Work out the finished part from the listing and answer in its coordinate system (mm). A direction names the side the tool comes from. Round coordinates to 2 decimals unless told otherwise and drop trailing zeros. Loops run counter-clockwise (first coordinate to the right, second up) from the corner with the lowest first, then second, coordinate; pieces in that order, holes last.
```python
from build123d import *

# Parameters (mm, degrees)
BASE_FLANGE1_DEPTH = 10
SKETCH6_R          = 2.5
CUT_EXTRUDE1_DEPTH = 35.932076949
SKETCH7_R          = 2
CUT_EXTRUDE2_DEPTH = 36.305806888


# Sheet-metal steps are written as plain solids
with BuildPart() as part:
    # Sketch1 → Base-Flange1 (new body)
    with BuildSketch(Plane.XY):
        with BuildLine():
            Line((0, 0), (13, 0))
            ThreePointArc((13, 0), (13.530330086, 0.219669914), (13.75, 0.75))
            Line((13.75, 0.75), (13.75, 5.75))
            ThreePointArc((13.75, 5.75), (14.409009742, 7.340990258), (16, 8))
            Line((16, 8), (32.5, 8))
            Line((32.5, 8), (32.5, 6.5))
            Line((32.5, 6.5), (16, 6.5))
            ThreePointArc((16, 6.5), (15.469669914, 6.280330086), (15.25, 5.75))
            Line((15.25, 5.75), (15.25, 0.75))
            ThreePointArc((15.25, 0.75), (14.590990258, -0.840990258), (13, -1.5))
            Line((13, -1.5), (0, -1.5))
            Line((0, -1.5), (0, 0))
        make_face()
    extrude(amount=BASE_FLANGE1_DEPTH)

    # Sketch6 → Cut-Extrude1 (cut, through all)
    with BuildSketch(Plane(origin=(0, 0, 0), x_dir=(1, 0, 0), z_dir=(0, 1, 0))):
        with Locations(Location((7.5, -5, 0), (0, 0, 270))):
            Circle(SKETCH6_R)
    extrude(amount=-CUT_EXTRUDE1_DEPTH, mode=Mode.SUBTRACT)

    # Sketch7 → Cut-Extrude2 (cut, through all)
    with BuildSketch(Plane(origin=(0, 8, 0), x_dir=(1, 0, 0), z_dir=(0, 1, 0))):
        with Locations(Location((27.5, -5, 0), (0, 0, 270))):
            Circle(SKETCH7_R)
    extrude(amount=-CUT_EXTRUDE2_DEPTH, mode=Mode.SUBTRACT)


solid = part.part
```
1. Consider probe 1 along Y at (x, z) = (9, 7.25); probe 2 along Y at (x, z) = (18.5, 0.5); probe 3 along X at (y, z) = (-0.5, 5). Determine where each line is inside the solid, lowest interval first.
Answer key:
probe 1: y = -1.5 to 0
probe 2: y = 6.5 to 8
probe 3: x = 0 to 5, 10 to 14.87
2. Determine the mould class of faces 1 (the face through (5.28, -0.74, 6.15)), 2 (the face through (15, 4, 10)), 3 (the face through (5, 0, 4)) for opening direction Z: +Z half, -Z half, draft (parallel to the pull), parting line (faces both ways), or undercut.
Answer key:
face 1: undercut
face 2: +Z half
face 3: draft
3. Find section A-A (z = 5). Write down the section's boundary in (x, y), then the cut area to 3 significant figures.
Answer key:
outline: (0, -1.5) - (5, -1.5) - (5, 0) - (0, 0) - close; (10, -1.5) - (13, -1.5) arc R2.25 ccw to (15.25, 0.75) - (15.25, 5.75) arc R0.75 cw to (16, 6.5) - (25.5, 6.5) - (25.5, 8) - (16, 8) arc R2.25 ccw to (13.75, 5.75) - (13.75, 0.75) arc R0.75 cw to (13, 0) - (10, 0) - close; (29.5, 6.5) - (32.5, 6.5) - (32.5, 8) - (29.5, 8) - close
area: 45.3 mm2
4. Given pin 1 (2 mm diameter, centred on y = 2.5, z = 6.5, fed in from -X); pin 2 (1 mm diameter, centred on y = 4.5, z = 8, fed in from +X); pin 3 (3 mm diameter, centred on x = 8.5, z = 3.5, fed in from +Y), each flat-ended and moving along its own axis, determine where each tip first touches the part or whether it passes through.
Answer key:
pin 1: stops at x = 13.75
pin 2: stops at x = 15.25
pin 3: stops at y = 0
5. Find section C-C (x = 24). Write down the section's boundary in (y, z), then the cut area to 3 significant figures.
Answer key:
outline: (6.5, 0) - (8, 0) - (8, 10) - (6.5, 10) - close
area: 15.0 mm2
6. Which of the six approach directions +Z, -Z, +X, -X, +Y, -Y give full straight-line access (tool end or side, diameter ignored) to faces 4 (the face through (24, 6.5, 5)), 5 (the face through (13.75, 3, 5)), 6 (the face through (0, -1, 5))?
Answer key:
face 4: +Z, -Z, +X, -Y
face 5: +Z, -Z, -X, +Y
face 6: +Z, -Z, -X, +Y, -Y
7. Find section D-D (y = 5). Write down the section's boundary in (x, z), then the cut area to 3 significant figures.
Answer key:
outline: (13.75, 0) - (15.25, 0) - (15.25, 10) - (13.75, 10) - close
area: 15.0 mm2
8. Find section B-B (x = 27.5). Write down the section's boundary in (y, z).
Answer key:
outline: (6.5, 0) - (8, 0) - (8, 3) - (6.5, 3) - close; (6.5, 7) - (8, 7) - (8, 10) - (6.5, 10) - close
